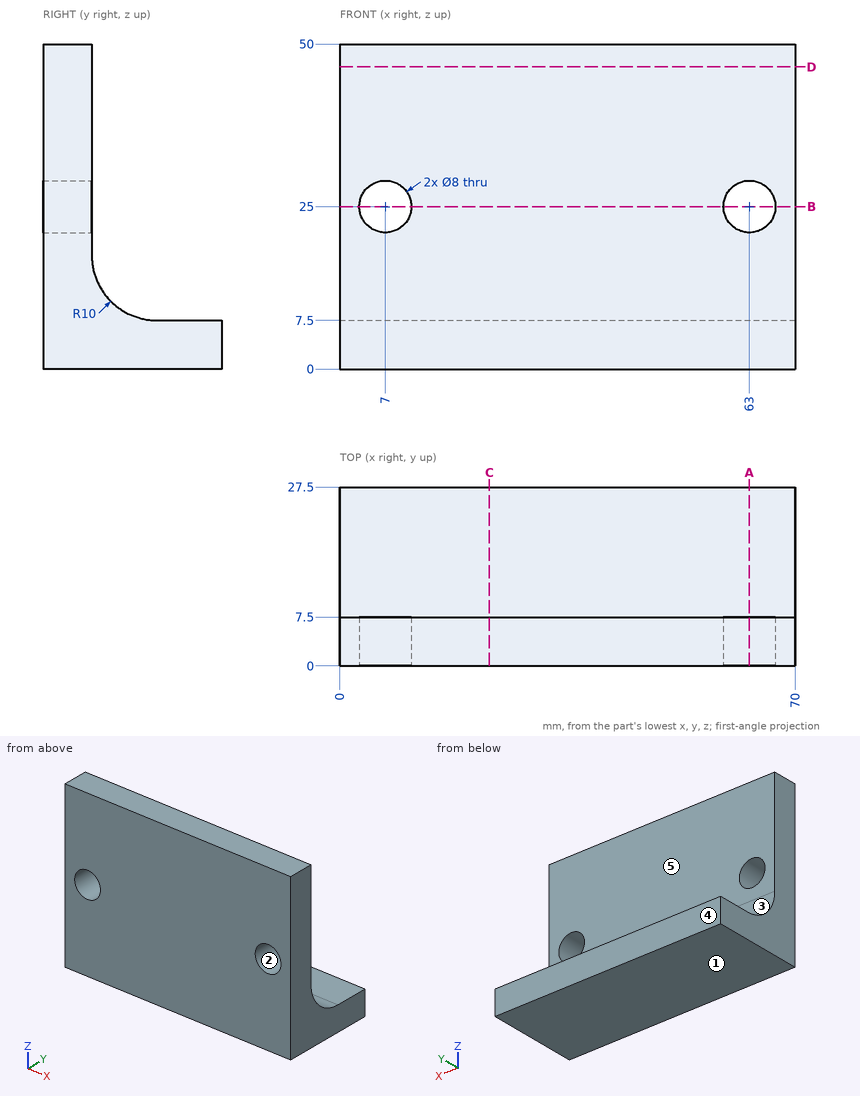
Input: dimensioned drawing with shaded views. Units: mm. Origin: part minimum x, y, z. A direction names the side the tool comes from. Round coordinates to 2 decimals unless told otherwise and drop trailing zeros. Loops run counter-clockwise (first coordinate to the right, second up) from the corner with the lowest first, then second, coordinate; pieces in that order, holes last.
1) Material intervals for line 1 (X direction, y = 3, z = 25); line 2 (Z direction, x = 7, y = 2.75); line 3 (Y direction, x = 64, z = 41.5), sorted ascending.
Ans:
line 1: x = 0 to 3, 11 to 59, 67 to 70
line 2: z = 0 to 21, 29 to 50
line 3: y = 0 to 7.5
2) Pull-direction query (Z, two-part tool) for the marked faces 1, 2 and 3; classes: released by +Z, released by -Z, zero draft, split by the parting line, or undercut.
Ans:
face 1: released by -Z
face 2: undercut
face 3: released by +Z
3) Section query A-A on x = 63. Return the cut outline in (y, z), plus the area to 3 significant figures.
Ans:
outline: (0, 0) - (27.5, 0) - (27.5, 7.5) - (17.5, 7.5) arc R10 cw to (7.5, 17.5) - (7.5, 21) - (0, 21) - close; (0, 29) - (7.5, 29) - (7.5, 50) - (0, 50) - close
area: 486 mm2
4) Section query D-D on z = 46.5. Return the cut outline in (x, y), plus the area to 3 significant figures.
Ans:
outline: (0, 0) - (70, 0) - (70, 7.5) - (0, 7.5) - close
area: 525 mm2
5) Section query B-B on z = 25. Return the cut outline in (x, y), plus the area to 3 significant figures.
Ans:
outline: (0, 0) - (3, 0) - (3, 7.5) - (0, 7.5) - close; (11, 0) - (59, 0) - (59, 7.5) - (11, 7.5) - close; (67, 0) - (70, 0) - (70, 7.5) - (67, 7.5) - close
area: 405 mm2
6) Set-up query: the marked faces 4 and 5. Return all of +Z, -Z, +X, -X, +Y, -Y with unobstructed straight access to the full face (end or side cutting, diameter ignored); none if empty.
Ans:
face 4: +Z, -Z, +X, -X, +Y
face 5: +Z, +X, -X, +Y
7) Section query C-C on x = 23. Return the cut outline in (y, z), plus the area to 3 significant figures.
Ans:
outline: (0, 0) - (27.5, 0) - (27.5, 7.5) - (17.5, 7.5) arc R10 cw to (7.5, 17.5) - (7.5, 50) - (0, 50) - close
area: 546 mm2
8) Pin query (flat end, axial travel): pin 1 (12 mm diameter, centred on x = 17, z = 42.5, fed in from +Y); pin 2 (5 mm diameter, centred on x = 27, y = 24.5, fed in from +Z). Return the tip coordinate at first contact, or that it passes through.
Ans:
pin 1: stops at y = 7.5
pin 2: stops at z = 7.5
